Geometry: see drawing. Coordinates: mm, zero at the bounding-box minimum. A direction names the side the tool comes from. Coordinates: 2 decimals unless noted, no trailing zeros. Loops run counter-clockwise (first coordinate to the right, second up) from the corner with the lowest first, then second, coordinate; pieces in that order, holes last. Notation, with made-up numbers: (-40, 12) -> (-20, 12) arc R34 cw to (-20, 51) -> close; hole circle Ø11 at (-16, 88.5). An arc over 180 degrees is marked (long way). One line per item, written item: value. Start each with the question number.
Item 1: Section query B-B on y = 15.24. Return loops of the section in (x, z) (1 decimal), then the cut area to 3 significant figures.
Item 2: Contact query for flat-ended pins moving along their axis: pin 1 Ø3 at (y, z) = (16, 5.5) entering from -X (1 decimal); pin 2 Ø4 at (y, z) = (14, 5.5) entering from -X; pin 3 Ø4.5 at (y, z) = (17, 8) entering from -X. Output: stop coordinate, or through.
Item 3: Section query C-C on y = 3.81. Return loops of the section in (x, z).
Item 4: Mould query, pull axis Z, two halves, no side actions, for the marked faces 3, 4 and 5. Classes: +Z half, -Z half, draft (parallel to the pull), parting line (faces both ways), or undercut.
Item 5: Set-up query: the marked faces 1 and 2. Return all of +Z, -Z, +X, -X, +Y, -Y with unobstructed straight access to the full face (end or side cutting, diameter ignored); none if empty.
Item 6: Ray query, probe 1 along Y at (x, z) = (3.81, 1.5) (1 decimal); probe 2 along Z at (x, y) = (5, 9) (1 decimal); probe 3 along X at (y, z) = (5.5, 1.25). Return the intervals inside material, ascending. Write a range as from..to.
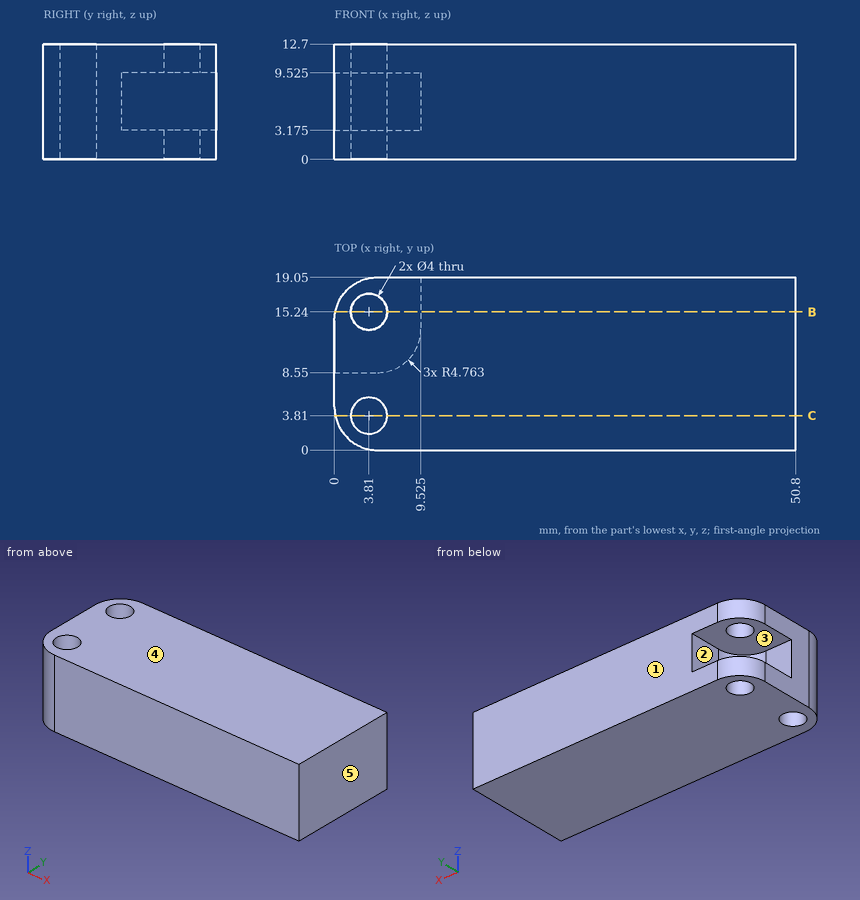
Reply:
1. outline: (0.1, 0) -> (1.8, 0) -> (1.8, 3.2) -> (0.1, 3.2) -> close; (0.1, 9.5) -> (1.8, 9.5) -> (1.8, 12.7) -> (0.1, 12.7) -> close; (5.8, 0) -> (50.8, 0) -> (50.8, 12.7) -> (5.8, 12.7) -> (5.8, 9.5) -> (9.5, 9.5) -> (9.5, 3.2) -> (5.8, 3.2) -> close
1. area: 559 mm²
2. pin 1: stops at x = 9.5
2. pin 2: stops at x = 9.34
2. pin 3: stops at x = 0.12
3. outline: (0.1, 0) -> (1.81, 0) -> (1.81, 12.7) -> (0.1, 12.7) -> close; (5.81, 0) -> (50.8, 0) -> (50.8, 12.7) -> (5.81, 12.7) -> close
4. face 3: undercut
4. face 4: +Z half
4. face 5: draft
5. face 1: +Z, -Z, +X, -X, +Y
5. face 2: -X, +Y
6. probe 1: y = 0.1..1.8, 5.8..13.2, 17.2..19
6. probe 2: z = 0..3.2, 9.5..12.7
6. probe 3: x = 0..2.74, 4.88..50.8
